Can you work these out from the model? Positions are in its coordinate system, mm. Face numbers are marked on the shaded views. A direction names the side the tool comes from. Round coordinates to 2 decimals unless told otherwise and drop trailing zeros. Write each loop counter-clockwise with the first axis right and the second up, starting at its lowest first coordinate (ties: lowest second). Pieces come first, ordered by that corner, then holes.
Q1. If we section it at D-D (y = 20.5): Please give me the cut outline in (x, z).
Q2. I'm going to push flat-ended pins straight in: pin 1 Ø2.5 at (y, z) = (3, 31.5) entering from -X; pin 2 Ø2.5 at (y, z) = (4, 34) entering from +X; pin 3 Ø0.8 at (x, y) = (8.5, 12.5) entering from +Z; pin 4 Ø2 at (y, z) = (4.5, 2) entering from -X. Where does each tip first touch, or does it pass through?
Q3. If we section it at B-B (z = 23): Please give me the cut outline in (x, y).
Q4. Please list where these lines run through material, in increasing order: line 1 along Z through (x, y) = (17, 7.25); line 2 along Z through (x, y) = (29, 20.5); line 3 along Z through (x, y) = (69, 2.5).
Q5. For the marked faces 1, 2, 3, 4 and 5, which set-ups out of +Z, -Z, +X, -X, +Y, -Y let a thin tool reach every point of the face, with its end or its side?
Q6. We'd pull the mould along X, two halves only. Please class the marked faces 6 and 7: +X half, -X half, draft (parallel to the pull), parting line (faces both ways), or undercut.
Q7. If we section it at C-C (x = 61): Please give me the cut outline in (y, z).
Q8. If we section it at A-A (x = 50): Please give me the cut outline in (y, z).
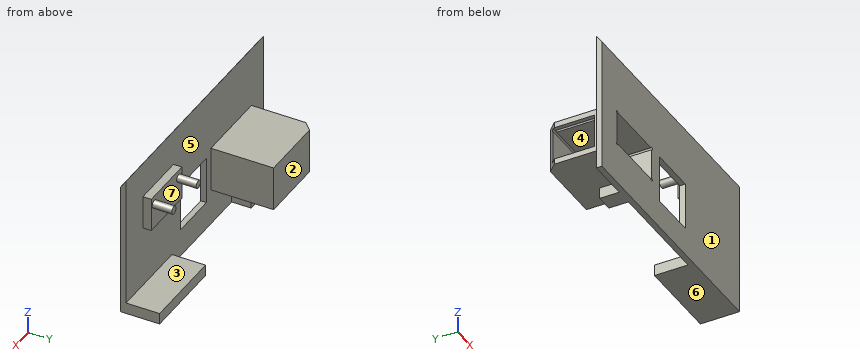
Solid Edge part; units mm, degrees
sketch "Sketch1" plane through (0, 0, 0) normal (0, -1, 0) x (1, 0, 0)
  line L0 (0, 50.6986) -> (13.1232, 65)
  line L1 (13.1232, 65) -> (90, 65)
  line L2 (90, 65) -> (90, 0)
  line L3 (90, 0) -> (0, 0)
  line L4 (0, 0) -> (0, 50.6986)
extrude "Protrusion1" add sketch "Sketch1" against normal blind 2
sketch "Sketch2" plane through (45, 0, 32.5) normal (0, -1, 0) x (1, 0, 0)
  line L0 (-35, -17.5) -> (-12.5, -17.5)
  line L1 (-12.5, -17.5) -> (-12.5, -5.5)
  line L2 (-12.5, -5.5) -> (-35, -5.5)
  line L3 (-35, -5.5) -> (-35, -17.5)
  dimension "D1" = 12.5
  dimension "D2" = 12.5
extrude "Cutout1" cut sketch "Sketch2" against normal through all
sketch "Sketch3" plane through (45, 2, 32.5) normal (0, 1, 0) x (-1, 0, 0)
  line L0 (12.5, -5.5) -> (35, -5.5)
  line L1 (35, -5.5) -> (35, -17.5)
  line L2 (35, -17.5) -> (12.5, -17.5)
  line L3 (12.5, -17.5) -> (12.5, -5.5)
  line L4 (10.5, -19.5) -> (37, -19.5)
  line L5 (37, -19.5) -> (37, -3.5)
  line L6 (37, -3.5) -> (10.5, -3.5)
  line L7 (10.5, -3.5) -> (10.5, -19.5)
extrude "Extrusionsausprägung_2" add sketch "Sketch3" along normal blind 20.4
sketch "Sketch4" plane through (24.25, 22.4, 21) normal (0, 1, 0) x (-1, 0, 0)
  line L0 (-10.25, 8) -> (16.25, 8)
  line L1 (16.25, 8) -> (16.25, -8)
  line L2 (16.25, -8) -> (-10.25, -8)
  line L3 (-10.25, -8) -> (-10.25, 8)
extrude "Extrusionsausprägung_3" add sketch "Sketch4" along normal blind 2
sketch "Sketch5" plane through (8, 13.2, 21) normal (-1, 0, 0) x (0, -1, 0)
  line L0 (-9.2, 6) -> (6.2, 6)
  line L1 (6.2, 6) -> (6.2, -6)
  line L2 (6.2, -6) -> (-9.2, -6)
  line L3 (-9.2, -6) -> (-9.2, 6)
extrude "Cutout2" cut sketch "Sketch5" against normal up to next
sketch "Sketch6" plane through (45, 0, 32.5) normal (0, -1, 0) x (1, 0, 0)
  arc A0 (-34.5, -5.5) -> (-35, -6) centre (-35, -5.5) ccw
  line L0 (-35, -5.5) -> (-35, -6)
  line L1 (-34.5, -5.5) -> (-35, -5.5)
  arc A1 (-13, -5.5) -> (-12.5, -6) centre (-12.5, -5.5) cw
  line L2 (-12.5, -5.5) -> (-12.5, -6)
  line L3 (-13, -5.5) -> (-12.5, -5.5)
  arc A2 (-12.5, -17) -> (-13, -17.5) centre (-12.5, -17.5) cw
  line L4 (-12.5, -17.5) -> (-13, -17.5)
  line L5 (-12.5, -17) -> (-12.5, -17.5)
  arc A3 (-34.5, -17.5) -> (-35, -17) centre (-35, -17.5) cw
  line L6 (-35, -17) -> (-35, -17.5)
  line L7 (-35, -17.5) -> (-34.5, -17.5)
  dimension "D1" = 34.5
extrude "Cutout3" cut sketch "Sketch6" against normal up to vertex (22.4 mm away)
sketch "Sketch7" plane through (8, 13.2, 21) normal (-1, 0, 0) x (0, -1, 0)
  arc A0 (-8.7, 6) -> (-9.2, 5.5) centre (-9.2, 6) ccw
  line L0 (-9.2, 6) -> (-9.2, 5.5)
  line L1 (-8.7, 6) -> (-9.2, 6)
  arc A1 (-9.2, -5.5) -> (-8.7, -6) centre (-9.2, -6) ccw
  line L2 (-9.2, -6) -> (-8.7, -6)
  line L3 (-9.2, -5.5) -> (-9.2, -6)
  dimension "D1" = 8.7
extrude "Cutout4" cut sketch "Sketch7" against normal up to vertex (24.5 mm away)
sketch "Sketch8" plane through (45, 2, 32.5) normal (0, 1, 0) x (-1, 0, 0)
  circle A0 centre (-32, 2.5) radius 1.4
  circle A1 centre (-16, 2.5) radius 1.4
extrude "Gy_521" add sketch "Sketch8" along normal blind 10
sketch "Sketch9" plane through (45, 2, 32.5) normal (0, 1, 0) x (-1, 0, 0)
  line L0 (-34, -6.5) -> (-14, -6.5)
  line L1 (-14, -6.5) -> (-14, 5.5)
  line L2 (-14, 5.5) -> (-34, 5.5)
  line L3 (-34, 5.5) -> (-34, -6.5)
  dimension "D1" = 34
  dimension "D2" = 14
extrude "Extrusionsausprägung_5" add sketch "Sketch9" along normal blind 3
chamfer "Fase_1" distance 3 angle 45 1 edges at (8, 24.4, 21)
sketch "Sketch10" plane through (45, 0, 32.5) normal (0, -1, 0) x (1, 0, 0)
  line L0 (-7.5, -5.5) -> (9.5, -5.5)
  line L1 (9.5, -5.5) -> (9.5, -22.5)
  line L2 (9.5, -22.5) -> (-7.5, -22.5)
  line L3 (-7.5, -22.5) -> (-7.5, -5.5)
  dimension "D1" = 7.5
extrude "Cutout5" cut sketch "Sketch10" against normal up to next
sketch "Sketch11" plane through (45, 0, 32.5) normal (0, -1, 0) x (1, 0, 0)
  line L0 (-45, 18.1986) -> (45, 18.1986)
extrude "Cutout6" cut sketch "Sketch11" against normal through all material side at (45, 0, 50.7486)
sketch "Sketch12" plane through (0, 1, 25.3493) normal (-1, 0, 0) x (0, 0, -1)
  line L0 (-25.3493, -1) -> (-22.4898, 1)
  line L1 (-22.4898, 1) -> (-25.3493, 1)
  line L2 (-25.3493, 1) -> (-25.3493, -1)
extrude "Cutout7" cut sketch "Sketch12" against normal through all
sketch "Sketch13" plane through (45, 2, 25.3493) normal (0, 1, 0) x (-1, 0, 0)
  line L0 (-45, -21.3493) -> (-15, -21.3493)
  line L1 (-15, -21.3493) -> (-15, -25.3493)
  line L2 (-15, -25.3493) -> (-45, -25.3493)
  line L3 (-45, -25.3493) -> (-45, -21.3493)
  dimension "D1" = 45
  dimension "D2" = 45
extrude "Extrusionsausprägung_6" add sketch "Sketch13" along normal blind 12
sketch "Sketch14" plane through (45, 2, 25.3493) normal (0, 1, 0) x (-1, 0, 0)
  line L0 (30, -25.3493) -> (24, -25.3493)
  line L1 (24, -25.3493) -> (24, -21.3493)
  line L2 (24, -21.3493) -> (30, -21.3493)
  line L3 (30, -21.3493) -> (30, -25.3493)
  dimension "D1" = 30
  dimension "D2" = 30
extrude "Extrusionsausprägung_7" add sketch "Sketch14" along normal blind 7
A:
1. outline: (8, 13) - (34.5, 13) - (34.5, 29) - (8, 29) - (8, 27) - (9.5, 27) arc R0.5 cw to (10.5, 27) - (32, 27) arc R0.5 cw (long way) to (32.5, 26.5) - (32.5, 15.5) arc R0.5 cw (long way) to (32, 15) - (10.5, 15) arc R0.5 cw to (9.5, 15) - (8, 15) - close
2. pin 1: stops at x = 0
2. pin 2: stops at x = 79
2. pin 3: stops at z = 29
2. pin 4: stops at x = 15
3. outline: (0, 0) - (10, 0) - (10, 7) - (8, 7) - (8, 2) - (0, 2) - close; (9, 22.4) - (32.5, 22.4) - (32.5, 0) - (37.5, 0) - (37.5, 2) - (34.5, 2) - (34.5, 24.4) - (11, 24.4) - close; (54.5, 0) - (90, 0) - (90, 2) - (54.5, 2) - close
4. line 1: z = 0 to 4, 13 to 15, 27 to 29
4. line 2: z = 13 to 15, 27 to 29
4. line 3: z = 0 to 4, 26 to 38
5. face 1: +Z, -Z, +X, -X, -Y
5. face 2: +Z, -Z, +X, -X, +Y
5. face 3: +X, -X, +Y
5. face 4: -Y
5. face 5: +Y
6. face 6: draft
6. face 7: undercut
7. outline: (0, 0) - (14, 0) - (14, 4) - (2, 4) - (2, 26) - (5, 26) - (5, 33.6) - (12, 33.6) - (12, 36.4) - (5, 36.4) - (5, 38) - (2, 38) - (2, 50.7) - (0, 47.84) - close
8. outline: (0, 0) - (2, 0) - (2, 10) - (0, 10) - close; (0, 27) - (2, 27) - (2, 50.7) - (0, 47.84) - close
